```python
from build123d import *

# Parameters (mm, degrees)
SKETCH1_W           = 57
SKETCH1_H           = 30
BOSS_EXTRUDE1_DEPTH = 5
SKETCH2_R           = 3.175
BOSS_EXTRUDE2_DEPTH = 4.5
SKETCH3_R           = 1.5367
CUT_EXTRUDE1_DEPTH  = 5
SKETCH4_R           = 12.85
SKETCH4_R_2         = 5.4
CUT_EXTRUDE2_DEPTH  = 2
SKETCH5_R           = 5
CUT_EXTRUDE3_DEPTH  = 10
SKETCH6_W           = 8
SKETCH6_H           = 30
BOSS_EXTRUDE3_DEPTH = 5
SKETCH7_R           = 5.4
SKETCH7_R_2         = 3.175
CUT_EXTRUDE4_DEPTH  = 0.5
SKETCH8_R           = 1.15
CUT_EXTRUDE5_DEPTH  = 15


with BuildPart() as part:
    # Sketch1 → Boss-Extrude1 (new body)
    with BuildSketch(Plane(origin=(0, 0, 0), x_dir=(1, 0, 0), z_dir=(0, 1, 0))):
        with Locations((6.5, 0)):
            Rectangle(SKETCH1_W, SKETCH1_H)
    extrude(amount=BOSS_EXTRUDE1_DEPTH)

    # Sketch2 → Boss-Extrude2 (add)
    with BuildSketch(Plane(origin=(0, 5, 0), x_dir=(1, 0, 0), z_dir=(0, 1, 0))):
        with Locations(Location((0, 0, 0), (0, 0, 270))):
            Circle(SKETCH2_R)
    extrude(amount=BOSS_EXTRUDE2_DEPTH)

    # Sketch3 → Cut-Extrude1 (cut)
    with BuildSketch(Plane(origin=(0, 5, 0), x_dir=(1, 0, 0), z_dir=(0, 1, 0))):
        with Locations(Location((-18, -11, 0), (0, 0, 270))):
            Circle(SKETCH3_R)
        with Locations(Location((18, 11, 0), (0, 0, 270))):
            Circle(SKETCH3_R)
    extrude(amount=-CUT_EXTRUDE1_DEPTH, mode=Mode.SUBTRACT)

    # Sketch4 → Cut-Extrude2 (cut)
    with BuildSketch(Plane(origin=(0, 5, 0), x_dir=(1, 0, 0), z_dir=(0, 1, 0))):
        with Locations(Location((0, 0, 0), (0, 0, 270))):
            Circle(SKETCH4_R)
        with Locations(Location((0, 0, 0), (0, 0, 270))):
            Circle(SKETCH4_R_2, mode=Mode.SUBTRACT)
    extrude(amount=-CUT_EXTRUDE2_DEPTH, mode=Mode.SUBTRACT)

    # Sketch5 → Cut-Extrude3 (cut)
    with BuildSketch(Plane(origin=(0, 5, 0), x_dir=(1, 0, 0), z_dir=(0, 1, 0))):
        with Locations(Location((19.6, 0, 0), (0, 0, 270))):
            Circle(SKETCH5_R)
    extrude(amount=-CUT_EXTRUDE3_DEPTH, mode=Mode.SUBTRACT)

    # Sketch6 → Boss-Extrude3 (add)
    with BuildSketch(Plane(origin=(0, 5, 0), x_dir=(1, 0, 0), z_dir=(0, 1, 0))):
        with Locations((39, 0)):
            Rectangle(SKETCH6_W, SKETCH6_H)
    extrude(amount=-BOSS_EXTRUDE3_DEPTH)

    # Sketch7 → Cut-Extrude4 (cut)
    with BuildSketch(Plane(origin=(0, 5, 0), x_dir=(1, 0, 0), z_dir=(0, 1, 0))):
        with Locations(Location((0, 0, 0), (0, 0, 270))):
            Circle(SKETCH7_R)
        with Locations(Location((0, 0, 0), (0, 0, 270))):
            Circle(SKETCH7_R_2, mode=Mode.SUBTRACT)
    extrude(amount=-CUT_EXTRUDE4_DEPTH, mode=Mode.SUBTRACT)

    # Sketch8 → Cut-Extrude5 (cut)
    with BuildSketch(Plane(origin=(0, 5, 0), x_dir=(1, 0, 0), z_dir=(0, 1, 0))):
        with Locations(Location((37.5, -8, 0), (0, 0, 270))):
            Circle(SKETCH8_R)
    extrude(amount=-CUT_EXTRUDE5_DEPTH, mode=Mode.SUBTRACT)


solid = part.part
```
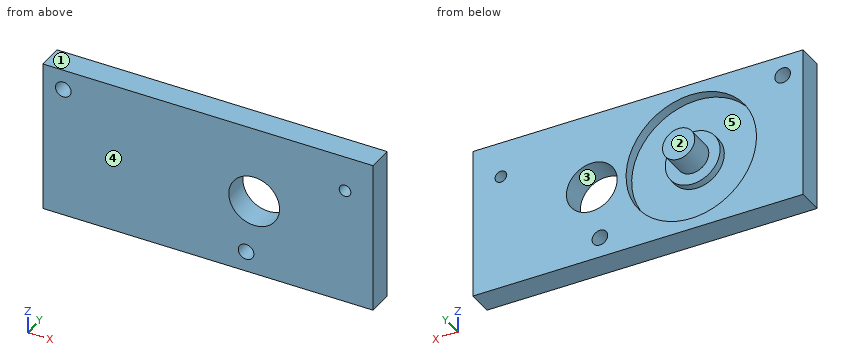
Read the model definition and answer for the solid it produces. Units are mm, in the model's axes. Face numbers are marked on the shaded views. A direction names the side the tool comes from. Give positions to 0.01 mm unless a question says otherwise; leave off trailing zeros. Write each loop counter-clockwise with the first axis right and the second up, starting at its lowest first coordinate (ties: lowest second). Pieces come first, ordered by that corner, then holes. Notation, with made-up numbers: (-7.75, -12) -> (27.25, -12) arc R12 cw to (27.25, 1) -> close; hole circle Ø1 at (40, 22.5). An arc over 180 degrees is marked (long way). Answer as a JSON object with one key per item and string values.
1) Section B-B on x = -18 is taken. Write down the section's boundary in (y, z), then the cut area to 3 significant figures.
Findings below:
{"outline": "(0, -15) -> (5, -15) -> (5, 9.46) -> (0, 9.46) -> close; (0, 12.54) -> (5, 12.54) -> (5, 15) -> (0, 15) -> close", "area": "135 mm^2"}
2) Straight lines are drawn through the part: probe 1 along X at (y, z) = (1, -11); probe 2 along X at (y, z) = (2.65, 8); probe 3 along X at (y, z) = (4.4, 0). For each, find the intervals that lie inside material, in ascending order. Write a range as from..to.
Findings below:
{"probe 1": "x = -22..16.46, 19.54..43", "probe 2": "x = -22..36.35, 38.65..43", "probe 3": "x = -22..-12.85, -5.4..5.4, 12.85..14.6, 24.6..43"}
3) Flat-ended cylindrical pins translate along their axes: pin 1 Ø4 at (x, z) = (-18, 11) entering from -Y; pin 2 Ø6 at (x, z) = (36.5, -7.5) entering from +Y. Find the tip coordinate at first contact, or state that the pin passes through.
Findings below:
{"pin 1": "stops at y = 0", "pin 2": "stops at y = 5"}
4) A tool of negligible diameter and unlimited length cuts with its end or side. For the marked faces 4 and 5, from which of +Z, -Z, +X, -X, +Y, -Y can it reach the whole face along a straight path? Write none if from no direction.
Findings below:
{"face 4": "+Z, -Z, +X, -X, -Y", "face 5": "+Y"}
5) Section C-C on y = 1.75 is taken. Write down the section's boundary in (x, z), then the cut area to 3 significant figures.
Findings below:
{"outline": "(-22, -15) -> (43, -15) -> (43, 15) -> (-22, 15) -> close; hole circle Ø3.07 at (-18, 11); hole circle Ø10 at (19.6, 0); hole circle Ø3.07 at (18, -11); hole circle Ø2.3 at (37.5, 8)", "area": "1,850 mm^2"}
6) Section A-A on z = 0 is taken. Write down the section's boundary in (x, y) (3 decimals), then the cut area to 3 significant figures.
Findings below:
{"outline": "(-22, 0) -> (14.6, 0) -> (14.6, 5) -> (12.85, 5) -> (12.85, 3) -> (5.4, 3) -> (5.4, 4.5) -> (3.175, 4.5) -> (3.175, 9.5) -> (-3.175, 9.5) -> (-3.175, 4.5) -> (-5.4, 4.5) -> (-5.4, 3) -> (-12.85, 3) -> (-12.85, 5) -> (-22, 5) -> close; (24.6, 0) -> (43, 0) -> (43, 5) -> (24.6, 5) -> close", "area": "272 mm^2"}
7) For a pull along Z with two mould halves and no side action, classify the marked faces 1, 2 and 3 as pulls with the +Z half, pulls with the -Z half, needs draft (parallel to the pull), parting line crosses it, or undercut.
Findings below:
{"face 1": "pulls with the +Z half", "face 2": "needs draft", "face 3": "undercut"}
8) Section D-D on x = 0 is taken. Write down the section's boundary in (y, z) (3 decimals), then the cut area to 3 significant figures.
Findings below:
{"outline": "(0, -15) -> (5, -15) -> (5, -12.85) -> (3, -12.85) -> (3, -5.4) -> (4.5, -5.4) -> (4.5, -3.175) -> (9.5, -3.175) -> (9.5, 3.175) -> (4.5, 3.175) -> (4.5, 5.4) -> (3, 5.4) -> (3, 12.85) -> (5, 12.85) -> (5, 15) -> (0, 15) -> close", "area": "147 mm^2"}
